Study the drawing (mm; zero at the part's minimum x, y, z) and answer. A direction names the side the tool comes from. Give positions to 0.01 mm unless a question says otherwise; leave off trailing zeros. Write each loop counter-clockwise with the first axis right and the second up, starting at its lowest first coordinate (ties: lowest second). Pieces come first, ordered by that corner, then holes.
1) Determine the mould class of the marked faces 1, 2 and 3 for opening direction Y: pulls with the +Y half, pulls with the -Y half, needs draft (parallel to the pull), parting line crosses it, or undercut.
2) A tool of negligible diameter and unlimited length cuts with its end or side. For the marked faces 4, 5 and 6, from which of +Z, -Z, +X, -X, +Y, -Y can it reach the whole face along a straight path? Write none if from no direction.
3) Given pin 1 Ø1 at (x, z) = (29.5, 13) entering from -Y; pin 2 Ø8 at (x, y) = (44.5, 5.5) entering from +Z; pin 3 Ø3 at (x, z) = (8, 3) entering from -Y; pin 4 Ø8 at (x, z) = (25.5, 13.5) entering from +Y, each flat-ended and moving along its own axis, determine where each tip first touches the part or whether it passes through.
4) Straight lines are drawn through the part: probe 1 along X at (y, z) = (18.5, 5.5) (1 decimal); probe 2 along Z at (x, y) = (50, 21); probe 3 along Y at (x, z) = (42, 1.5). For each, find the intervals that lie inside material, in ascending order.
5) Find section D-D (z = 3.25). Count the separate pieces of the cut face and the enclosed holes in it, plus the area to 3 significant figures.
6) Find section A-A (y = 7). Determine the outline of the cut face in (x, z) (1 decimal).
7) Find section C-C (y = 18). Determine the outline of the cut face in (x, z) (1 decimal).
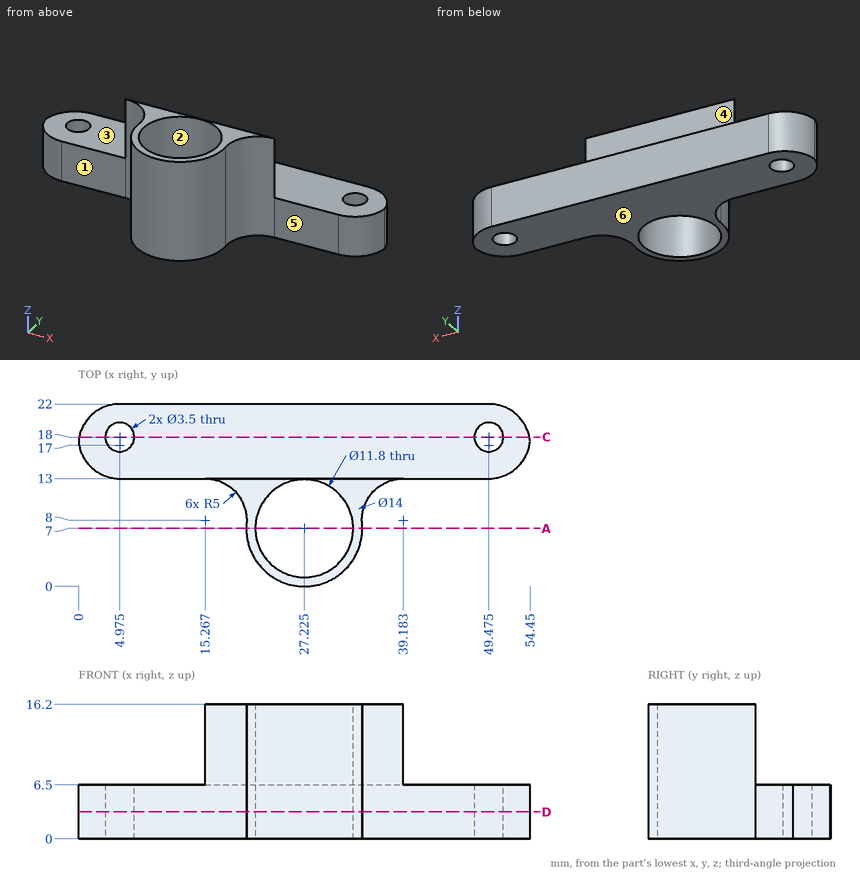
Results:
1. face 1: pulls with the -Y half
1. face 2: undercut
1. face 3: needs draft
2. face 4: +Z, +X, -X, +Y
2. face 5: +Z, -Z, +X, -Y
2. face 6: -Z, +X, -X, +Y, -Y
3. pin 1: stops at y = 0.23
3. pin 2: passes through
3. pin 3: stops at y = 13
3. pin 4: stops at y = 13
4. probe 1: x = 0.2 to 3.3, 6.7 to 47.8, 51.2 to 54.2
4. probe 2: z = 0 to 6.5
4. probe 3: y = 13 to 22
5. separate pieces: 1
5. enclosed holes: 3
5. area: 512 mm2
6. outline: (20.2, 0) - (21.3, 0) - (21.3, 16.2) - (20.2, 16.2) - close; (33.1, 0) - (34.2, 0) - (34.2, 16.2) - (33.1, 16.2) - close
7. outline: (0.1, 0) - (3.2, 0) - (3.2, 6.5) - (0.1, 6.5) - close; (6.7, 0) - (47.7, 0) - (47.7, 6.5) - (6.7, 6.5) - close; (51.2, 0) - (54.4, 0) - (54.4, 6.5) - (51.2, 6.5) - close
